Verification items for the finished model (mm, model axes). A direction names the side the tool comes from. Give positions to 0.01 mm unless a question says otherwise; leave off trailing zeros. Loops run counter-clockwise (first coordinate to the right, second up) from the corner with the lowest first, then second, coordinate; pieces in that order, holes last. Notation, with made-up numbers: M 1.25,71 L 18.25,71 A30 ccw 18.25,96 Z; hole C -11,16 d7. An arc over 180 degrees is marked long. Use a Markdown table: item, result.
Autodesk Inventor part; units mm, degrees
ref_plane "YZ Plane" through (0, 0, 0) normal (1, 0, 0) x (0, 1, 0)
ref_plane "XZ Plane" through (0, 0, 0) normal (0, 1, 0) x (-1, 0, 0)
ref_plane "XY Plane" through (0, 0, 0) normal (0, 0, 1) x (1, 0, 0)
sketch "스케치1" plane through (0, 0, 0) normal (0, 0, 1) x (1, 0, 0)
  line L0 (0, 0) -> (0, -10)
  line L1 (0, -10) -> (75.7735, -10)
  line L2 (0, 0) -> (70, 0)
  line L3 (0, 0) -> (70, 0) construction
  line L4 (70, 0) -> (95, 43.3013)
  line L5 (95, 43.3013) -> (138.3013, 18.3013)
  line L6 (138.3013, 18.3013) -> (133.3013, 9.641)
  line L7 (133.3013, 9.641) -> (98.6603, 29.641)
  line L8 (98.6603, 29.641) -> (75.7735, -10)
  dimension "d0" = 10
  dimension "d10" = 70
  dimension "d12" = 50
  dimension "d13" = 120
  dimension "d14" = 50
  dimension "d15" = 90
  dimension "d16" = 10
  dimension "d17" = 90
  dimension "d18" = 10
extrude "돌출1" add sketch "스케치1" along normal mid plane 60
fillet "모깎기1" radius 10 2 edges at (0, -5, 30) (0, -5, -30)
fillet "모깎기2" radius 20 2 edges at (135.8013, 13.9711, 30) (135.8013, 13.9711, -30)
fillet "모깎기3" radius 5 1 edges at (75.7735, -10, 0)
fillet "모깎기4" radius 3 1 edges at (98.6603, 29.641, 0)
sketch "스케치2" plane through (70, 0, 30) normal (0, 1, 0) x (1, 0, 0)
  line L0 (-45, 30) -> (-25, 30) construction
  line L1 (-45, 24) -> (-25, 24)
  line L2 (-25, 36) -> (-45, 36)
  arc A0 (-45, 36) -> (-45, 24) centre (-45, 30) ccw
  arc A1 (-25, 24) -> (-25, 36) centre (-25, 30) ccw
  line L3 (-70, 10) -> (-70, 50)
  line L4 (0, 0) -> (-60, 0)
  point P0 (-70, 30)
  point P1 (-35, 30)
  dimension "d23" = 12
  dimension "d24" = 20
  dimension "d25" = 25
  dimension "d26" = 30
extrude "돌출2" cut sketch "스케치2" against normal blind 60
sketch "스케치3" plane through (95, 43.3013, 30) normal (0.5, 0.866, 0) x (0.866, -0.5, 0)
  circle A0 centre (25, 30) radius 12
  circle A1 centre (25, 51) radius 3
  circle A2 centre (25, 9) radius 3
  line L0 (0, 60) -> (0, 0)
  line L1 (0, 60) -> (30, 60)
  point P0 (-60.6218, 30)
  dimension "d29" = 24
  dimension "d30" = 6
  dimension "d32" = 6
  dimension "d33" = 21
  dimension "d34" = 21
  dimension "d36" = 25
  dimension "d37" = 25
  dimension "d38" = 30
extrude "돌출3" cut sketch "스케치3" against normal blind 60
properties part number "1번"
(1) Cross-section at B-B on y = -5. Record the cut outline in (x, z), then the cut area to 3 significant figures.
Results below:
| item | result |
|---|---|
| outline | M 0,-20 A10 ccw 10,-30 L 78.66,-30 L 78.66,30 L 10,30 A10 ccw 0,20 Z; hole M 25,-6 L 45,-6 A6 ccw 45,6 L 25,6 A6 ccw Z |
| area | 4,320 mm^2 |
(2) Gauge pin test, flat ends, axial feed: P1, Ø1, axis at y = 17.5, z = 6, coming from the +X side; P2, Ø3, axis at x = 109, z = -15.5, coming from the -Y side; P3, Ø5, axis at y = 29, z = -18.5, coming from the +X side. Record the tip position at first contact, or that the pin passes through.
Results below:
| item | result |
|---|---|
| P1 | x = 138.13 |
| P2 | y = 22.81 |
| P3 | x = 124.1 |
(3) Cross-section at D-D on x = 60. Record the cut outline in (y, z).
Results below:
| item | result |
|---|---|
| outline | M -10,-30 L 0,-30 L 0,30 L -10,30 Z |
(4) Material ranges on line 1 (X direction, y = 26.5, z = -21.5); line 2 (X direction, y = 14, z = 16.5); line 3 (Y direction, x = 65, z = 7), recorded low to high.
Results below:
| item | result |
|---|---|
| line 1 | 85.3 to 96.85, 104.1 to 110.75, 117.58 to 124.1 |
| line 2 | 78.08 to 89.63, 125.75 to 134.56 |
| line 3 | -10 to 0 |
(5) Draft check along X on faces 6 (the flat face through (82.325, 21.348, -0.42)), 7 (the flat face through (35, -5, -6)), 8 (the flat face through (135.836, 14.032, -0.14)), 9 (the flat face through (36, -10, -7)). Enter one of: +X half, -X half, draft (parallel to the pull), parting line (faces both ways), or undercut.
Results below:
| item | result |
|---|---|
| face 6 | -X half |
| face 7 | undercut |
| face 8 | +X half |
| face 9 | draft |
(6) Cross-section at A-A on x = 29.5. Record the cut outline in (y, z), then the cut area to 3 significant figures.
Results below:
| item | result |
|---|---|
| outline | M -10,-30 L 0,-30 L 0,-6 L -10,-6 Z; M -10,6 L 0,6 L 0,30 L -10,30 Z |
| area | 480 mm^2 |
(7) Set-up check for faces 1 (the flat face through (73, 3, -30)), 2 (the flat face through (87.328, 10.013, -0.42)), 3 (the cylindrical face through (116.664, 25.101, -21.901)), 4 (the cylindrical face through (19, -5, 0)), 5 (the flat face through (35, 0, -7)): record each of +Z, -Z, +X, -X, +Y, -Y from which the full face is reachable in a straight line by a thin tool's end or side.
Results below:
| item | result |
|---|---|
| face 1 | -Z, +X, -X, +Y, -Y |
| face 2 | +Z, -Z, -Y |
| face 3 | none |
| face 4 | +Y, -Y |
| face 5 | +Z, -Z, -X, +Y |
(8) Cross-section at C-C on z = -14. Record the cut outline in (x, y), then the cut area to 3 significant figures.
Results below:
| item | result |
|---|---|
| outline | M 0,-10 L 72.89,-10 A5 ccw 77.22,-7.5 L 97.16,27.04 A3 cw 101.26,28.14 L 132.95,9.84 L 137.95,18.5 L 95,43.3 L 70,0 L 0,0 Z |
| area | 1,650 mm^2 |
